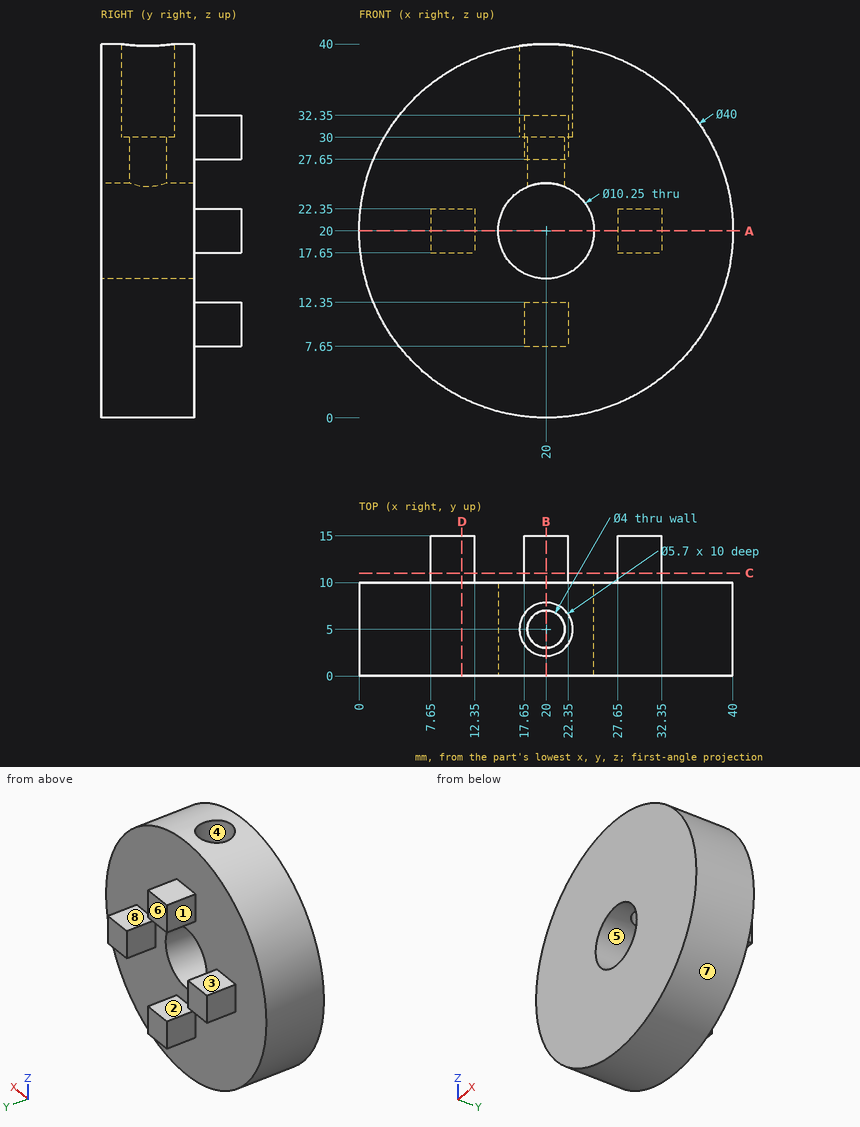
Can you work these out from the drawing? Everything is in mm from the part's minimum corner. A direction names the side the tool comes from. Give positions to 0.01 mm unless a question says otherwise; leave off trailing zeros. Loops run counter-clockwise (first coordinate to the right, second up) from the corner with the lowest first, then second, coordinate; pieces in that order, holes last. Notation, with made-up numbers: M -33,48.5 L 16,48.5 A12 ccw 16,54.5 Z; hole C -30,58 d5. An arc over 180 degrees is marked long. Put each result on its own line as item: value. Start each with the question number.
(1) I want a section at C-C on y = 11. Please give me the cut outline in (x, z), then the cut area to 3 significant figures.
(2) Will these pins go through, and if not, where does the flat tip stop? pin 1 Ø1.5 at (x, y) = (30.5, 2.5) entering from +Z; pin 2 Ø2.5 at (x, y) = (19.5, 11.5) entering from +Z; pin 3 Ø3.5 at (x, y) = (20, 5) entering from -Z; pin 4 Ø8 at (x, z) = (20, 34) entering from +Y.
(3) If we mould it in two halves opening along Z, with no side actions, what happens to the marked faces 5, 6, 7 and 8? For each: +Z half, -Z half, draft (parallel to the pull), parting line (faces both ways), or undercut.
(4) I want a section at B-B on x = 20. Please give me the cut outline in (y, z) (3 decimals).
(5) I want a section at A-A on z = 20. Please give me the cut outline in (x, y) (3 decimals), then the cut area to 4 significant figures.
(6) For the marked faces 1, 2, 3 and 4, which set-ups out of +Z, -Z, +X, -X, +Y, -Y let a thin tool reach every point of the face, with its end or its side?
(7) I need wall thicknesses on line 1 along Y through (x, z) = (20, 37); line 2 along Y through (x, z) = (9, 10); line 3 along Z through (x, y) = (15.5, 0.5). Which ranges of each line are inside material? Lowest first, please. Write a range as [from, to].
(8) I want a section at D-D on x = 11. Please give me the cut outline in (y, z), then the cut area to 3 significant figures.
Answer block:
1. outline: M 7.65,17.65 L 12.35,17.65 L 12.35,22.35 L 7.65,22.35 Z; M 17.65,7.65 L 22.35,7.65 L 22.35,12.35 L 17.65,12.35 Z; M 17.65,27.65 L 22.35,27.65 L 22.35,32.35 L 17.65,32.35 Z; M 27.65,17.65 L 32.35,17.65 L 32.35,22.35 L 27.65,22.35 Z
1. area: 88.4 mm^2
2. pin 1: z = 37.46
2. pin 2: z = 32.35
2. pin 3: z = 0
2. pin 4: y = 15
3. face 5: undercut
3. face 6: draft
3. face 7: parting line
3. face 8: +Z half
4. outline: M 0,0 L 10,0 L 10,7.65 L 15,7.65 L 15,12.35 L 10,12.35 L 10,14.875 L 0,14.875 Z; M 0,25.125 L 3,25.125 L 3,30 L 2.15,30 L 2.15,40 L 0,40 Z; M 7,25.125 L 10,25.125 L 10,27.65 L 15,27.65 L 15,32.35 L 10,32.35 L 10,40 L 7.85,40 L 7.85,30 L 7,30 Z
5. outline: M 0,0 L 14.875,0 L 14.875,10 L 12.35,10 L 12.35,15 L 7.65,15 L 7.65,10 L 0,10 Z; M 25.125,0 L 40,0 L 40,10 L 32.35,10 L 32.35,15 L 27.65,15 L 27.65,10 L 25.125,10 Z
5. area: 344.5 mm^2
6. face 1: +Z, -Z, -X, +Y
6. face 2: +X, -X, +Y
6. face 3: +Z, +X, -X, +Y
6. face 4: +Z
7. line 1: [0, 2.15], [7.85, 10]
7. line 2: [0, 10]
7. line 3: [0.51, 17.55], [22.45, 39.49]
8. outline: M 0,2.14 L 10,2.14 L 10,17.65 L 15,17.65 L 15,22.35 L 10,22.35 L 10,37.86 L 0,37.86 Z
8. area: 381 mm^2
